from build123d import *

# Parameters (mm, degrees)
SKETCH_1_W           = 150
SKETCH_1_H           = 15
EXTRUDE_1_DEPTH      = 8
FILLET_1_R           = 5
SKETCH_6_R           = 12.5
EXTRUDE_2_DEPTH      = 8
SKETCH_11_R          = 1
CUT_EXTRUDE_8_DEPTH  = 10
EXTRUDE_5_DEPTH      = 10
EXTRUDE_5_DEPTH_BACK = 57
SKETCH_15_R          = 3
CUT_EXTRUDE_9_REACH  = 163.707
SKETCH_16_R          = 1


with BuildPart() as part:
    # 草图1 → 凸台-拉伸1 (new body)
    with BuildSketch(Plane(origin=(0, 0, 0), x_dir=(0, 0, -1), z_dir=(1, 0, 0))):
        with Locations((75, 7.5)):
            Rectangle(SKETCH_1_W, SKETCH_1_H)
    extrude(amount=EXTRUDE_1_DEPTH)

    # 圆角1
    fillet_1_edges = [part.edges().sort_by_distance(p)[0] for p in [
        (4, 15, 0),
        (4, 15, -150),
        (4, 0, -150),
        (4, 0, 0),
    ]]
    fillet(fillet_1_edges, radius=FILLET_1_R)

    # 草图6 → 凸台-拉伸2 (add)
    with BuildSketch(Plane(origin=(8, 0, 0), x_dir=(0, 0, -1), z_dir=(1, 0, 0))):
        with Locations((6.4, 7.5)):
            Circle(SKETCH_6_R)
    extrude(amount=-EXTRUDE_2_DEPTH)

    # 草图11 → 切除-拉伸8 (cut)
    with BuildSketch(Plane.ZY):
        with Locations((-145, 7.5)):
            Circle(SKETCH_11_R)
        with Locations((-135, 7.5)):
            Circle(SKETCH_11_R)
        with Locations((85, 7.5)):
            Circle(SKETCH_11_R)
        with Locations((95, 7.5)):
            Circle(SKETCH_11_R)
    extrude(amount=-CUT_EXTRUDE_8_DEPTH, mode=Mode.SUBTRACT)

    # 草图15 → 凸台-拉伸5 (add, two sides: drawn at the far end of the back side and taken through both)
    with BuildSketch(Plane.ZY.offset(-EXTRUDE_5_DEPTH_BACK)):
        with Locations((-6.4, 7.5)):
            Circle(SKETCH_15_R)
    extrude(amount=EXTRUDE_5_DEPTH + EXTRUDE_5_DEPTH_BACK)

    # 草图16 → 切除-拉伸9 (cut, up to next)
    with BuildSketch(Plane.XY, mode=Mode.PRIVATE) as cut_extrude_9_sk1:
        with Locations((-7, 7.5)):
            Circle(SKETCH_16_R)
    cut_extrude_9_tool1 = extrude(cut_extrude_9_sk1.sketch, amount=-CUT_EXTRUDE_9_REACH, mode=Mode.PRIVATE) & part.part
    # 草图16 → 切除-拉伸9 (cut, up to next)
    with BuildSketch(Plane.XY, mode=Mode.PRIVATE) as cut_extrude_9_sk2:
        with Locations((54, 7.5)):
            Circle(SKETCH_16_R)
    cut_extrude_9_tool2 = extrude(cut_extrude_9_sk2.sketch, amount=-CUT_EXTRUDE_9_REACH, mode=Mode.PRIVATE) & part.part
    add(cut_extrude_9_tool1.solids().sort_by_distance((-7, 7.5, 0))[0], mode=Mode.SUBTRACT)
    add(cut_extrude_9_tool2.solids().sort_by_distance((54, 7.5, 0))[0], mode=Mode.SUBTRACT)


solid = part.part
Input: part model. Units: mm. Frame: model coordinates. A direction names the side the tool comes from. Coordinates: 2 decimals unless noted, no trailing zeros. Write each loop counter-clockwise with the first axis right and the second up, starting at its lowest first coordinate (ties: lowest second). Pieces come first, ordered by that corner, then holes. Notation, with made-up numbers: M 50.25,63 L 92.25,63 A38 ccw 92.25,101 Z; hole C -36.5,15 d7. An arc over 180 degrees is marked long. Answer as a JSON object with one key per item and string values. Group by question number.
(1) Ray query, line 1 along X through (y, z) = (7.5, -7); line 2 along Y through (x, z) = (5.75, -135); line 3 along X through (y, z) = (5.25, -58). Return the intervals inside material, ascending. Write a range as [from, to].
(2) Contact query for flat-ended pins moving along their axis: P1, Ø8, axis at x = 49, y = 10.5, coming from the -Z side; P2, Ø7.5, axis at y = 10.5, z = -110, coming from the +X side; P3, Ø9, axis at x = 5.5, z = -109, coming from the +Y side; P4, Ø5, axis at x = 12, z = -74, coming from the +Y side. Output: stop coordinate, or through.
(3) Set-up query: faces 1 (the face through (4, 0, -80)), 2 (the face through (32.84, 8.4, -3.54)), 3 (the face through (-4.93, 6.35, -3.63)), 4 (the face through (4, 15, -80)), 5 (the face through (57, 8, -6)). Return all of +Z, -Z, +X, -X, +Y, -Y with unobstructed straight access to the full face (end or side cutting, diameter ignored); none if empty.
(4) Section B-B on x = 35. Output: boundary loops of the cut face in (y, z), plus the area to 3 significant figures.
(5) Section D-D on z = -51. Output: boundary loops of the cut face in (x, y), plus the area to 3 significant figures.
(6) Section A-A on z = -6.4. Output: boundary loops of the cut face in (x, y).
(7) Section C-C on y = 17.5. Output: boundary loops of the cut face in (x, z).
Result set:
{
 "1": {"line 1": "x = [-10, -8], [-6, 53], [55, 57]", "line 2": "y = [0, 6.5], [8.5, 15]", "line 3": "x = [0, 8]"},
 "2": {"P1": "stops at z = -9.4", "P2": "stops at x = 8", "P3": "stops at y = 15", "P4": "passes through"},
 "3": {"face 1": "-Z, +X, -X, -Y", "face 2": "+X", "face 3": "-X", "face 4": "-Z, +X, -X, +Y", "face 5": "+Z, -Z, +X, +Y, -Y"},
 "4": {"outline": "C 7.5,-6.4 d6", "area": "28.3 mm2"},
 "5": {"outline": "M 0,0 L 8,0 L 8,15 L 0,15 Z", "area": "120 mm2"},
 "6": {"outline": "M -10,4.5 L 0,4.5 L 0,-5 L 8,-5 L 8,4.5 L 57,4.5 L 57,10.5 L 8,10.5 L 8,20 L 0,20 L 0,10.5 L -10,10.5 Z; hole C -7,7.5 d2; hole C 54,7.5 d2"},
 "7": {"outline": "M 0,-13.9 L 8,-13.9 L 8,1.1 L 0,1.1 Z"}
}
